```python
from build123d import *

# Parameters (mm, degrees)
F0_W     = 100
F0_H     = 50
F1_DEPTH = 25
F2_R     = 10
F3_DEPTH = 25.001
F5_DEPTH = 25


with BuildPart() as f1:
    # F0 (on Top) → F1 (new body)
    with BuildSketch(Plane.XY):
        with Locations((42.712342, 58.077995)):
            Rectangle(F0_W, F0_H)
    extrude(amount=F1_DEPTH)

    # F2 (on face) → F3 (cut, through all)
    with BuildSketch(Plane.XY.offset(25)):
        with Locations((16.594408, 52.342981)):
            Circle(F2_R)
    extrude(amount=-F3_DEPTH, mode=Mode.SUBTRACT)

    # F4 (on face) → F5 (join)
    with BuildSketch(Plane(origin=(0, 0, 0), x_dir=(1, 0, 0), z_dir=(0, 0, -1))):
        Polygon((45.338004, -47.928774), (60.75959, -78.947715), (79.911988, -50.082759), align=None)
    extrude(amount=F5_DEPTH)


solid = f1.part
```
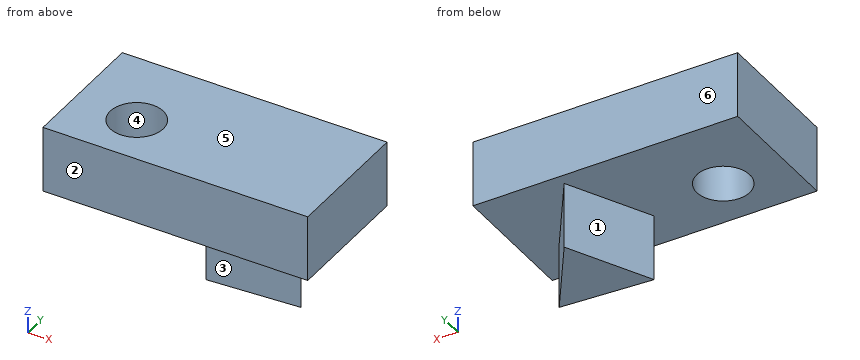
For this review, take the finished solid that the model builds, in its own axes (mm). Face numbers are marked on the shaded views. A direction names the side the tool comes from. Coordinates: 2 decimals unless noted, no trailing zeros. Loops run counter-clockwise (first coordinate to the right, second up) from the corner with the lowest first, then second, coordinate; pieces in that order, holes last.
1. Mouldability with a two-part tool opening along Y and no side actions: class the marked faces 3, 4, 5 and 6 as +Y half, -Y half, draft (parallel to the pull), parting line (faces both ways), or undercut.
2. For the marked faces 1 and 2, list the 3-axis set-ups (+Z, -Z, +X, -X, +Y, -Y) from which the entire face can be reached by the end or side of a thin tool; tool diameter is ignored.
3. Insertion check: P1, Ø2, axis at y = 59.5, z = -19, coming from the -X side; P2, Ø4, axis at y = 64.5, z = -6.5, coming from the -X side. Each pin has a flat end and moves straight along its axis. Give the tip position at first contact, or say it passes through.
4. Add section D-D, the plane y = 76.5. Give the boundary of the cut face in (x, z).
5. Add section A-A, the plane y = 58.5. Give the boundary of the cut face in (x, z), then the cut area to 3 significant figures.
6. For line 1 (Z direction, x = 31.5, y = 71); line 2 (Y direction, x = 15.5, z = 3.5); line 3 (X direction, y = 46, z = 13.5), list the stretches that pass through material, from the lowest coordinate up.
7. Add section C-C, the plane z = 6.5. Give the boundary of the cut face in (x, y), then the cut area to 3 significant figures.
8. Add section B-B, the plane x = 23.5. Give the boundary of the cut face in (y, z).
Result:
1. face 3: -Y half
1. face 4: undercut
1. face 5: draft
1. face 6: +Y half
2. face 1: -Z, -X, +Y
2. face 2: +Z, -Z, +X, -X, -Y
3. P1: stops at x = 50.59
3. P2: stops at x = 52.58
4. outline: (-7.29, 0) - (59.54, 0) - (59.54, -25) - (62.38, -25) - (62.38, 0) - (92.71, 0) - (92.71, 25) - (-7.29, 25) - close
5. outline: (-7.29, 0) - (8.71, 0) - (8.71, 25) - (-7.29, 25) - close; (24.47, 0) - (50.59, 0) - (50.59, -25) - (74.33, -25) - (74.33, 0) - (92.71, 0) - (92.71, 25) - (24.47, 25) - close
5. area: 2,700 mm2
6. line 1: z = 0 to 25
6. line 2: y = 33.08 to 42.4, 62.28 to 83.08
6. line 3: x = -7.29 to 8.86, 24.33 to 92.71
7. outline: (-7.29, 33.08) - (92.71, 33.08) - (92.71, 83.08) - (-7.29, 83.08) - close; hole circle Ø20 at (16.59, 52.34)
7. area: 4,690 mm2
8. outline: (33.08, 0) - (45.11, 0) - (45.11, 25) - (33.08, 25) - close; (59.58, 0) - (83.08, 0) - (83.08, 25) - (59.58, 25) - close
